```python
from build123d import *

# Parameters (mm, degrees)
CYLINDER002001001002003_R           = 4
CYLINDER002001001002003_DEPTH       = 2
BOX001002001003003_W                = 15
BOX001002001003003_H                = 13
BOX001002001003003_DEPTH            = 6
BOX001001001_W                      = 15
BOX001001001_H                      = 13
BOX001001001_DEPTH                  = 6
BOX001002001003002_W                = 70
BOX001002001003002_H                = 40
BOX001002001003002_DEPTH            = 22
CYLINDER002001001002002_R           = 11
CYLINDER002001001002002_DEPTH       = 70
CYLINDER002001001002002_PITCH_ANGLE = 90
CYLINDER001_R                       = 11
CYLINDER001_DEPTH                   = 70
CYLINDER001_PITCH_ANGLE             = 90


with BuildPart() as powerbutton:
    # Cylinder002001001002003 → Cylinder002001001002003 (new body)
    with BuildSketch(Plane(origin=(16, 20, 10), x_dir=(1, 0, 0), z_dir=(0, 0, 1))):
        Circle(CYLINDER002001001002003_R)
    extrude(amount=CYLINDER002001001002003_DEPTH)


with BuildPart() as usb1:
    # Box001002001003003 → Box001002001003003 (new body)
    with BuildSketch(Plane(origin=(60, 13.5, -1), x_dir=(1, 0, 0), z_dir=(0, 0, 1))):
        with Locations((7.5, 6.5)):
            Rectangle(BOX001002001003003_W, BOX001002001003003_H)
    extrude(amount=BOX001002001003003_DEPTH)


with BuildPart() as fusion001001:
    # Box001001001 → Box001001001 (new body)
    with BuildSketch(Plane(origin=(60, 13.5, -10), x_dir=(1, 0, 0), z_dir=(0, 0, 1))):
        with Locations((7.5, 6.5)):
            Rectangle(BOX001001001_W, BOX001001001_H)
    extrude(amount=BOX001001001_DEPTH)

    # Fusion001001: union PowerButton, USB1
    add(powerbutton.part)
    add(usb1.part)


with BuildPart() as box001002001003002:
    # Box001002001003002 → Box001002001003002 (new body)
    with BuildSketch(Plane.XY.offset(-11)):
        with Locations((35, 20)):
            Rectangle(BOX001002001003002_W, BOX001002001003002_H)
    extrude(amount=BOX001002001003002_DEPTH)


with BuildPart() as cylinder002001001002002:
    # Cylinder002001001002002 → Cylinder002001001002002 (new body)
    with BuildSketch(Plane.XY):
        Circle(CYLINDER002001001002002_R)
    extrude(amount=CYLINDER002001001002002_DEPTH)


with BuildPart() as cylinder002001001002002_1:
    # Cylinder002001001002002 pitch: moved
    add(cylinder002001001002002.part.rotate(Axis((0, 0, 0), (0, 1, 0)), CYLINDER002001001002002_PITCH_ANGLE))


with BuildPart() as cylinder002001001002002_2:
    # Cylinder002001001002002 placement: moved
    add(cylinder002001001002002_1.part)


with BuildPart() as obj1:
    # Cylinder001 → Cylinder001 (new body)
    with BuildSketch(Plane.XY):
        Circle(CYLINDER001_R)
    extrude(amount=CYLINDER001_DEPTH)


with BuildPart() as obj1_1:
    # Cylinder001 pitch: moved
    add(obj1.part.rotate(Axis((0, 0, 0), (0, 1, 0)), CYLINDER001_PITCH_ANGLE))


with BuildPart() as obj1_2:
    # Cylinder001 placement: moved
    add(obj1_1.part.moved(Location((0, 40, 0))))

    # Fusion002001002002002001002: union Box001002001003002, Cylinder002001001002002
    add(box001002001003002.part)
    add(cylinder002001001002002_2.part)

    # Cut: cut Fusion001001
    add(fusion001001.part, mode=Mode.SUBTRACT)


with BuildPart() as obj1_3:
    # Cut placement: moved
    add(obj1_2.part.moved(Location((70, 10, 19))))


solid = obj1_3.part
```
Can you work these out from the model? Positions are in its coordinate system, mm. A direction names the side the tool comes from. Coordinates: 2 decimals unless noted, no trailing zeros. Write each loop counter-clockwise with the first axis right and the second up, starting at its lowest first coordinate (ties: lowest second). Pieces come first, ordered by that corner, then holes. Notation, with made-up numbers: M 38.25,43 L 96.25,43 A21 ccw 96.25,70 Z; hole C -1,-34 d1. An arc over 180 degrees is marked long. Write item = value, one per line. Start each with the question number.
Q1. Thinking about a two-plate mould opening in Z: for faces 4 (the face through (135, 36.5, 12)), 5 (the face through (86, 30, 29)), 6 (the face through (70, 30, 19)), which applies, released by +Z, released by -Z, zero draft, split by the parting line, or undercut?
Q2. If I drill on L1, parallel to Z at x = 133, y = 28; L2, parallel to X at y = 30, z = 29.2; L3, parallel to X at y = 30.5, z = 19, over which ranges is the centre line in solid material (lowest first)? Write a range as [from, to].
Q3. On a 3-axis mill with a long thin cutter (end or side, diameter ignored), from which of +Z, -Z, +X, -X, +Y, -Y can I reach the whole of each face in a straight line? I mean faces 1 (the face through (140, 30, 16)), 2 (the face through (85.479, 33.966, 29.493)), 3 (the face through (130, 30, 21)). Say none if no direction works.
Q4. I'm going to push flat-ended pins straight in: pin 1 (3 mm diameter, centred on x = 134.5, z = 12.5, fed in from +Y); pin 2 (5 mm diameter, centred on x = 137.5, z = 11, fed in from -Y); pin 3 (2 mm diameter, centred on x = 80, y = 53, fed in from +Z); pin 4 (6.5 mm diameter, centred on y = 29, z = 12.5, fed in from +X). Where does each tip first touch, or does it pass through?
Q5. If we section it at C-C, the plane y = 30: Write out the boundary of the cut face in (x, z), then the cut area to 3 significant figures.
Q6. If we section it at D-D, the plane x = 86: Write out the boundary of the cut face in (y, z), then the cut area to 3 significant figures.
Q7. If we section it at B-B, the plane x = 132: Write out the boundary of the cut face in (y, z).
Q8. If we section it at A-A, the plane z = 19: Write out the boundary of the cut face in (x, y), then the cut area to 3 significant figures.
Check sheet entries:
q1.face_4 = undercut
q1.face_5 = released by +Z
q1.face_6 = zero draft
q2.L1 = [8, 9], [15, 18], [24, 30]
q2.L2 = [70, 82], [90, 140]
q2.L3 = [70, 130]
q3.face_1 = +Z, -Z, +X, +Y, -Y
q3.face_2 = +Z
q3.face_3 = +X
q4.pin_1 = 59.8
q4.pin_2 = 0.47
q4.pin_3 = 29.82
q4.pin_4 = 140
q5.outline = M 70,8 L 140,8 L 140,9 L 130,9 L 130,15 L 140,15 L 140,18 L 130,18 L 130,24 L 140,24 L 140,30 L 90,30 L 90,29 L 82,29 L 82,30 L 70,30 Z
q5.area = 1,410 mm²
q6.outline = M 10,8 L 50,8 A11 ccw 50,30 L 34,30 L 34,29 L 26,29 L 26,30 L 10,30 A11 ccw Z
q6.area = 1,250 mm²
q7.outline = M 10,8 L 50,8 A11 ccw 50,30 L 10,30 A11 ccw Z; hole M 23.5,9 L 36.5,9 L 36.5,15 L 23.5,15 Z; hole M 23.5,18 L 36.5,18 L 36.5,24 L 23.5,24 Z
q8.outline = M 70,-1 L 140,-1 L 140,23.5 L 130,23.5 L 130,36.5 L 140,36.5 L 140,61 L 70,61 Z
q8.area = 4,210 mm²
